The figure shows three views and two pictorial views of one solid part (mm, origin at its lowest corner). Answer the questions. A direction names the side the tool comes from. Coordinates: 2 decimals unless noted, no trailing zeros. Write each loop counter-clockwise with the first axis right and the second up, starting at its lowest first coordinate (ties: lowest second). Pieces come first, ordered by that corner, then holes. Notation, with made-up numbers: (6, 77) - (22, 77) arc R25 cw to (22, 95) - close; hole circle Ø10 at (85, 61). An arc over 180 degrees is marked (long way). Use a Markdown table: item, result. Add a question column.
(1) Given pin 1 Ø6 at (x, y) = (20, 7) entering from -Z; pin 2 Ø10 at (y, z) = (8, 13.5) entering from +X; pin 3 Ø1.5 at (y, z) = (16, 17) entering from -X; pin 4 Ø6 at (x, z) = (26.5, 7.5) entering from -Y, each flat-ended and moving along its own axis, determine where each tip first touches the part or whether it passes through.
(2) The part is cut by section C-C, the plane x = 23. Give the vertices of the cut face in (y, z).
(3) Find the intervals of material crossed by line 1 (Y direction, x = 15, z = 8.25); line 2 (Z direction, x = 12.5, y = 12); line 3 (Y direction, x = 22, z = 15), in increasing order. Write a range as from..to.
(4) For a pull along X with two mould halves and no side action, classify the marked faces 3 and 4 as released by +X, released by -X, zero draft, split by the parting line, or undercut.
(5) A tool of negligible diameter and unlimited length cuts with its end or side. For the marked faces 1 and 2, from which of +Z, -Z, +X, -X, +Y, -Y can it reach the whole face along a straight path? Write none if from no direction.
(6) The part is cut by section B-B, the plane y = 15. Give the vertices of the cut face in (x, z), then the cut area to 3 significant figures.
(7) The part is cut by section D-D, the plane y = 10. Give the vertices of the cut face in (x, z), then the cut area to 3 significant figures.
(8) The part is cut by section A-A, the plane z = 4. Give the vertices of the cut face in (x, y), then the cut area to 3 significant figures.
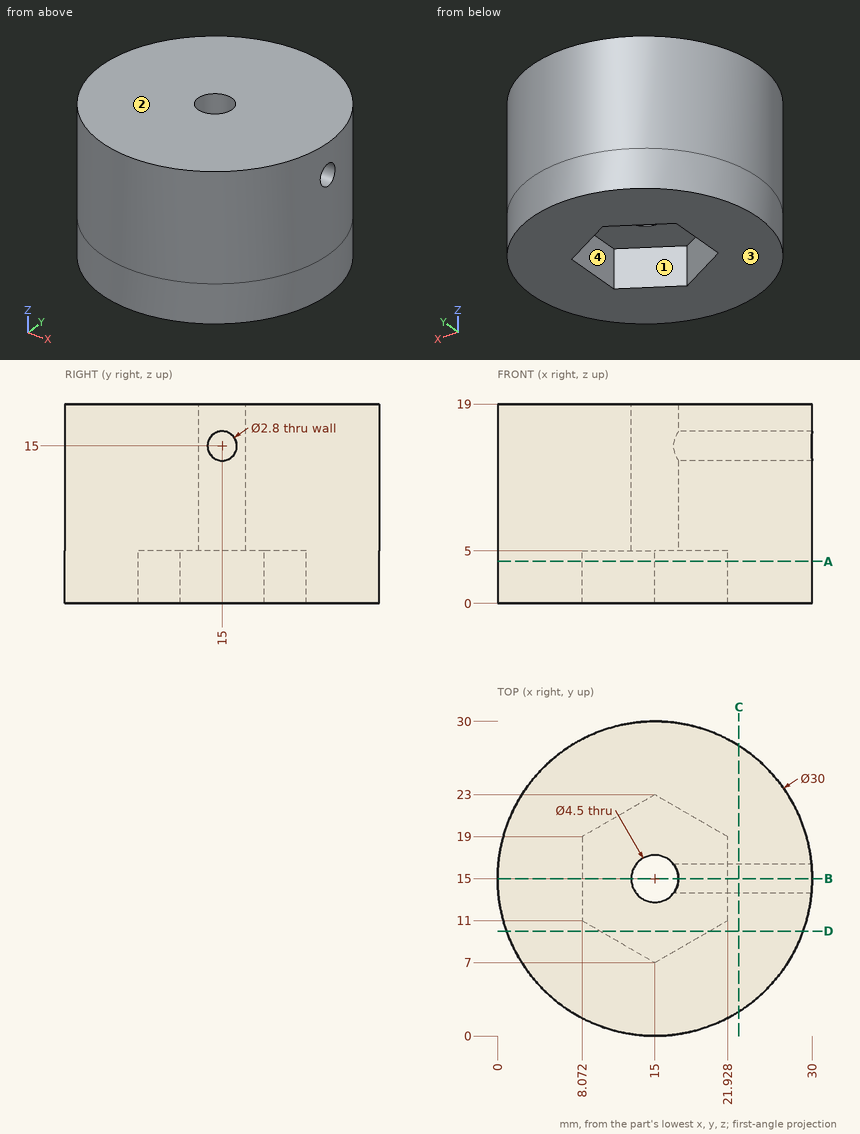
Model answer:
| question | item | result |
|---|---|---|
| 1 | pin 1 | z = 0 |
| 1 | pin 2 | x = 29.87 |
| 1 | pin 3 | x = 0 |
| 1 | pin 4 | y = 2.64 |
| 2 | outline | (2.31, 0) - (27.69, 0) - (27.69, 19) - (2.31, 19) - close; hole circle Ø2.8 at (15, 15) |
| 3 | line 1 | 0..12.75, 17.25..30 |
| 3 | line 2 | 5..19 |
| 3 | line 3 | 1.73..13.6, 16.4..28.27 |
| 4 | face 3 | zero draft |
| 4 | face 4 | undercut |
| 5 | face 1 | -Z |
| 5 | face 2 | +Z, +X, -X, +Y, -Y |
| 6 | outline | (0, 0) - (8.07, 0) - (8.07, 5) - (12.75, 5) - (12.75, 19) - (0, 19) - close; (17.25, 5) - (21.93, 5) - (21.93, 0) - (30, 0) - (30, 13.6) - (17.25, 13.6) - close; (17.25, 16.4) - (30, 16.4) - (30, 19) - (17.25, 19) - close |
| 6 | area | 402 mm^2 |
| 7 | outline | (0.86, 0) - (9.8, 0) - (9.8, 5) - (20.2, 5) - (20.2, 0) - (29.14, 0) - (29.14, 19) - (0.86, 19) - close |
| 7 | area | 485 mm^2 |
| 8 | outline | circle Ø30 at (15, 15); hole (8.07, 11) - (15, 7) - (21.93, 11) - (21.93, 19) - (15, 23) - (8.07, 19) - close |
| 8 | area | 541 mm^2 |
